Source: three-view drawing plus pictorial views. Frame: mm from the lowest corner of the part. Give positions to 0.01 mm unless a question says otherwise; leave off trailing zeros. Loops run counter-clockwise (first coordinate to the right, second up) from the corner with the lowest first, then second, coordinate; pieces in that order, holes last.
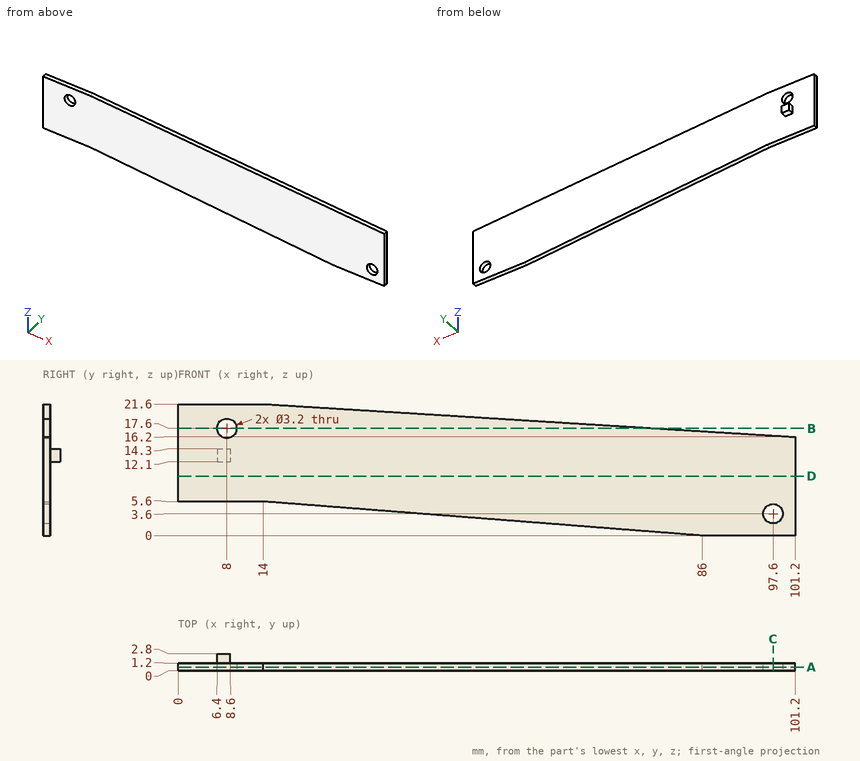
1) Cut plane B-B (z = 17.6). Return loops of the section in (x, y).
Checks:
outline: (0, 0) - (6.4, 0) - (6.4, 1.2) - (0, 1.2) - close; (9.6, 0) - (78.59, 0) - (78.59, 1.2) - (9.6, 1.2) - close
2) Cut plane C-C (x = 97.6). Return loops of the section in (y, z), and give its area (3 significant figures).
Checks:
outline: (0, 0) - (1.2, 0) - (1.2, 2) - (0, 2) - close; (0, 5.2) - (1.2, 5.2) - (1.2, 16.42) - (0, 16.42) - close
area: 15.9 mm2
3) Cut plane A-A (y = 0.6). Return loops of the section in (x, z).
Checks:
outline: (0, 5.6) - (14, 5.6) - (86, 0) - (101.2, 0) - (101.2, 16.2) - (14, 21.6) - (0, 21.6) - close; hole circle Ø3.2 at (8, 17.6); hole circle Ø3.2 at (97.6, 3.6)
4) Cut plane D-D (z = 9.75). Return loops of the section in (x, y), and give its area (3 significant figures).
Checks:
outline: (0, 0) - (101.2, 0) - (101.2, 1.2) - (0, 1.2) - close
area: 121 mm2
5) Ray query, probe 1 along Z at (x, y) = (8, 0.7); probe 2 along Y at (x, z) = (87, 13.5); probe 3 along X at (y, z) = (1.85, 13). Return the intervals inside material, ascending.
Checks:
probe 1: z = 5.6 to 16, 19.2 to 21.6
probe 2: y = 0 to 1.2
probe 3: x = 6.4 to 8.6
6) Contact query for flat-ended pins moving along their axis: P1, Ø4, axis at x = 8, z = 17.6, coming from the +Y side; P2, Ø0.5, axis at x = 7, y = 2.5, coming from the -Z side; P3, Ø1.9, axis at x = 97.6, z = 3.6, coming from the +Y side; P4, Ø0.8, axis at y = 2, z = 12.5, coming from the +X side. Output: stop coordinate, or through.
Checks:
P1: stops at y = 1.2
P2: stops at z = 12.1
P3: passes through
P4: stops at x = 8.6
